Autodesk Inventor part; units mm, degrees
ref_plane "YZ Plane" through (0, 0, 0) normal (1, 0, 0) x (0, 1, 0)
ref_plane "XZ Plane" through (0, 0, 0) normal (0, 1, 0) x (-1, 0, 0)
ref_plane "XY Plane" through (0, 0, 0) normal (0, 0, 1) x (1, 0, 0)
sketch "Sketch1" plane through (0, 0, 0) normal (1, 0, 0) x (0, 1, 0)
  line L0 (-0.0645, -0.0614) -> (-0.0645, 12.6386) construction
  line L1 (-0.0645, 12.6386) -> (-0.0645, 25.3386) construction
  line L2 (-0.0645, -0.0614) -> (33.5905, -0.0614) construction
  line L3 (-0.0645, -0.0614) -> (33.5814, 17.8149) construction
  line L4 (33.5814, 17.8149) -> (33.5814, 30.5149) construction
  line L5 (33.5814, 30.5149) -> (33.5814, 43.2149) construction
  line L6 (-0.0645, -0.0614) -> (-0.0645, -25.4614) construction
  line L7 (-0.0645, -25.4614) -> (-0.0645, -50.8614) construction
  line L8 (-0.0645, -50.8614) -> (-0.0645, -88.9614) construction
  line L9 (-0.0645, -88.9614) -> (-0.0645, -127.0614) construction
  line L10 (-0.0645, -127.0614) -> (33.5905, -127.0614) construction
  line L11 (-0.0645, -127.0614) -> (33.5905, -144.9206) construction
  line L12 (-0.0645, -50.8614) -> (33.5905, -50.8614) construction
  line L13 (-0.0645, -50.8614) -> (33.5905, -68.7206) construction
  line L14 (33.5905, -68.7206) -> (33.5905, -81.4206) construction
  line L15 (33.5905, -81.4206) -> (33.5905, -94.1206) construction
  line L16 (33.5905, -144.9206) -> (33.5905, -106.8206) construction
  line L17 (33.5905, -106.8206) -> (96.5027, -106.8206) construction
  line L18 (33.5905, -144.9206) -> (56.4857, -106.8206) construction
  line L19 (33.5905, -68.7206) -> (56.4857, -106.8206) construction
  line L20 (-0.0645, -50.8614) -> (-0.0645, -63.5614) construction
  line L21 (-0.0645, -63.5614) -> (-0.0645, -76.2614) construction
  line L22 (33.5905, -0.0614) -> (67.2455, -0.0614) construction
  line L23 (67.2455, -0.0614) -> (33.5814, 17.8149) construction
  line L24 (67.2455, -0.0614) -> (67.2455, 25.3386) construction
  line L25 (67.2455, 25.3386) -> (67.2455, 25.3386) construction
  line L26 (67.2455, 25.3386) -> (73.5955, 25.3386) construction
  line L27 (67.2455, 25.3386) -> (60.8955, 25.3386) construction
  line L28 (-19.1145, -0.0711) -> (-19.1145, -127.0711)
  line L29 (-19.1145, -0.0711) -> (-19.1145, 32.0046)
  line L30 (-19.1145, 63.4289) -> (18.9855, 63.4289) construction
  line L31 (39.9379, -190.511) -> (19.05, -190.5323)
  line L32 (-19.05, -190.571) -> (-19.0726, -168.346) construction
  line L33 (-19.1145, 63.4289) -> (18.9855, 63.4289)
  line L34 (-19.1145, 63.4289) -> (-19.1145, 41.2039) construction
  line L35 (-19.05, -190.571) -> (-19.0726, -168.346)
  line L36 (-19.05, -190.571) -> (19.05, -190.5323) construction
  arc A0 (-11.2228, -178.4175) -> (19.05, -190.5323) centre (19.0055, -146.7627) ccw
  arc A1 (18.9855, 63.4289) -> (-10.4946, 51.0726) centre (22.5956, 13.4704) ccw
  line L37 (-19.1145, 41.2039) -> (-19.1145, 63.4289)
  line L38 (-19.081, -160.0737) -> (-19.1145, -127.0711)
  line L39 (19.05, -190.5323) -> (-19.05, -190.571)
  arc A2 (-10.4946, 51.0726) -> (-19.1145, 32.0046) centre (6.2855, 32.0046) ccw
  arc A3 (-19.081, -160.0737) -> (-11.2228, -178.4175) centre (6.319, -160.0479) ccw
  line L40 (82.55, -43.1133) -> (82.55, -47.5335)
  line L41 (82.55, -190.4677) -> (82.55, -154.3842)
  line L42 (82.55, 3.175) -> (82.55, 63.4289)
  line L43 (82.55, 63.4289) -> (18.9855, 63.4289)
  line L44 (19.05, -190.5323) -> (50.8, -190.5)
  line L45 (82.55, -190.4677) -> (82.55, -117.4427)
  arc A4 (59.4372, -181.357) -> (82.55, -117.4427) centre (-17.378, -117.4427) ccw
  arc A5 (39.9379, -190.511) -> (59.4372, -181.357) centre (39.9121, -165.1111) ccw
  line L46 (82.55, 63.4289) -> (82.55, -38.1711)
  line L47 (82.55, 63.4289) -> (114.3, 63.4289)
  line L48 (120.65, 57.0789) -> (120.65, 15.7647)
  arc A6 (108.6074, -5.8395) -> (95.5578, -16.5987) centre (141.4695, -58.9906) ccw
  arc A7 (84.9949, -32.2402) -> (82.55, -43.1133) centre (107.95, -43.1133) ccw
  arc A8 (108.6074, -5.8395) -> (120.65, 15.7647) centre (95.25, 15.7647) ccw
  arc A9 (120.65, 57.0789) -> (114.3, 63.4289) centre (114.3, 57.0789) ccw
  line L49 (82.55, -190.4677) -> (82.55, -79.4019)
  line L50 (82.55, -63.4677) -> (84.1375, -63.4677)
  line L51 (82.55, -117.4427) -> (82.55, -134.9348)
  line L52 (82.55, -117.4427) -> (82.55, -113.6327)
  line L53 (82.55, -63.4677) -> (88.9, -63.4677)
  line L54 (82.55, -63.4677) -> (82.55, -76.1677)
  line L55 (82.55, -63.4677) -> (82.55, -50.7677)
  arc A10 (88.9, -63.4677) -> (84.7021, -52.298) centre (76.3064, -61.827) ccw
  arc A11 (82.55, -47.5335) -> (84.7021, -52.298) centre (88.9, -47.5335) ccw
  arc A12 (84.7021, -74.6374) -> (82.55, -79.4019) centre (88.9, -79.4019) ccw
  line L56 (82.55, -63.4677) -> (84.1375, -63.4677)
  line L57 (84.1375, -63.4677) -> (84.1375, -139.6677)
  line L58 (82.55, -117.4427) -> (95.25, -139.6677)
  line L59 (95.25, -139.6677) -> (75.6405, -153.9552)
  line L60 (82.55, -63.4677) -> (77.47, -63.4677)
  line L61 (77.47, -63.4677) -> (77.47, -85.6927)
  line L62 (88.9, -63.4677) -> (88.9, -139.0447)
  line L63 (88.9, -63.4677) -> (88.8195, -33.8988)
  arc A13 (95.5578, -16.5987) -> (88.8195, -33.8988) centre (114.2194, -33.8296) ccw
  line L64 (33.5905, -144.9206) -> (48.1955, -144.9206)
  line L65 (48.1955, -144.9206) -> (48.1955, -119.5206)
  arc A14 (39.9379, -190.511) -> (88.9, -139.0447) centre (37.3696, -139.0447) ccw
  line L66 (84.1375, -139.6677) -> (48.1955, -139.6677)
  line L67 (48.1955, -139.6677) -> (48.1955, -119.5206)
  point P0 (82.55, -106.8206)
  point P1 (120.65, 63.4289)
  point P2 (120.65, -0.0711)
  point P3 (82.55, -148.9209)
  point P4 (88.7962, -25.3679)
  point P5 (88.8909, -60.1177)
  point P6 (44.795, -190.0373)
  dimension "d81" = 33.655
  dimension "d82" = 38.1
  dimension "d86" = 12.7
  dimension "d93" = 25.4
  dimension "d94" = 38.1
  dimension "d95" = 38.1
  dimension "d98" = 33.655
  dimension "d109" = 38.1
  dimension "d110" = 12.7
  dimension "d111" = 12.7
  dimension "d112" = 38.1
  dimension "d113" = 44.45
  dimension "d114" = 12.7
  dimension "d115" = 12.7
  dimension "d116" = 33.655
  dimension "d117" = 25.4
  dimension "d118" = 0
  dimension "d119" = 6.35
  dimension "d120" = 6.35
  dimension "d122" = 19.05
  dimension "d126" = 127
  dimension "d127" = 63.5
  dimension "d129" = 38.1
  dimension "d130" = 22.225
  dimension "d131" = 22.225
  dimension "d132" = 38.1
  dimension "d133" = 50.0888
  dimension "d134" = 25.4
  dimension "d135" = 25.4
  dimension "d137" = 31.75
  dimension "d138" = 73.025
  dimension "d139" = 25.4
  dimension "d140" = 101.6
  dimension "d141" = 38.1
  dimension "d142" = 25.4
  dimension "d143" = 6.35
  dimension "d144" = 62.4897
  dimension "d145" = 127
  dimension "d153" = 6.35
  dimension "d154" = 12.7
  dimension "d155" = 12.7
  dimension "d157" = 12.7
  dimension "d158" = 6.35
  dimension "d159" = 1.5875
  dimension "d160" = 76.2
  dimension "d161" = 5.08
  dimension "d162" = 22.225
  dimension "d163" = 38.1
  dimension "d164" = 25.4
  dimension "d166" = 25.4
extrude "Extrusion1" add sketch "Sketch1" along normal blind 1.5875 contours L29 A2 A1 L43 L47 A9 L48 A8 A6 A13 L63 L53 L57 A12 L49 A4 A5 A14 L31 A0 A3 L38 L28 | A5 A4 L59 L45 L41 A14 | L41 L45 L59 A14 | A4 L66 L45 L59 | L59 L45 L66 L57 L58 L62 A14 | A4 L45 L66 | L58 L57 L66 L45 | L49 A12 L57 L58 | L58 L57 L53 L62 | L63 A10
hole "Hole4" at (0, -0.0645, -0.0614) at (0, -0.0645, 12.6386) at (0, -0.0645, 25.3386) at (0, -0.0645, -127.0614) at (0, 33.5905, -144.9206) at (0, -0.0645, -50.8614) at (0, 33.5814, 43.2149) at (0, 33.5814, 30.5149) at (0, 33.5814, 17.8149) at (0, 33.5905, -68.7206) at (0, 33.5905, -81.4206) at (0, 33.5905, -94.1206) at (0, -0.0645, -63.5614) at (0, -0.0645, -76.2614) at (0, 56.4857, -106.8206) at (0, 60.8955, 25.3386) at (0, 73.5955, 25.3386) at (0, 48.1955, -119.5206) at (0, 84.1375, -63.4677) at (0, 77.47, -85.6927) at (0, 84.1375, -139.6677) direction (1, 0, 0) diameter 4.7625 end through all
properties part number "dtplate"
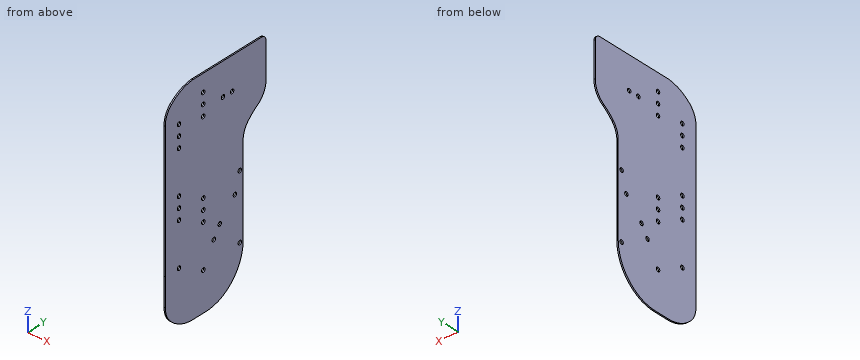
CAD build for the part. Positions are in the model's coordinates, mm. Give positions to 0.01 mm unless a question says otherwise; leave off trailing zeros. Order: outer loops, then holes, each group sorted by start corner. A loop starts at its lowest first (then second) coordinate and runs counter-clockwise, first axis right, second up. Notation, with made-up numbers: M 13.5,80 L 57.5,80 A18 cw 57.5,107 Z; hole C -14,-39 d8. An arc over 180 degrees is marked long. Put each result on its own line as item: value. Start each with the question number.
(1) Flat gauge pin, fed straight in: pin 1 Ø3 at (y, z) = (60.9, 25.34) entering from -X. Where does the tip first touch, or does it go through?
(2) Saw through at D-D, the plane z = -172. Write the cut outline in (x, y), then the cut area to 3 significant figures.
(3) Saw through at B-B, the plane y = 91.5. Write the cut outline in (x, z), then the cut area to 3 significant figures.
(4) Saw through at A-A, the plane z = 0. Write the cut outline in (x, y), then the cut area to 3 significant figures.
(5) Saw through at C-C, the plane x = 0.3. Give the number of separate pieces and of enclosed holes in the cut face, then the cut area to 3 significant figures.
(6) Drill centre lines: line 1 along Y through (x, z) = (1.15, 25); line 2 along Y through (x, z) = (1.2, -38); line 3 along Y through (x, z) = (1.2, 13). Where is each one in solid material? Low to high.
Check result:
1. pin 1: passes through
2. outline: M 0,-16.09 L 1.59,-16.09 L 1.59,76.98 L 0,76.98 Z
2. area: 148 mm2
3. outline: M 0,-22.47 L 1.59,-22.47 L 1.59,63.43 L 0,63.43 Z
3. area: 136 mm2
4. outline: M 0,-19.11 L 1.59,-19.11 L 1.59,-2.44 L 0,-2.44 Z; M 0,2.32 L 1.59,2.32 L 1.59,115.17 L 0,115.17 Z
4. area: 206 mm2
5. separate pieces: 1
5. enclosed holes: 21
5. area: 28,200 mm2
6. line 1: y = -19.11 to -2.42, 2.29 to 58.54, 63.25 to 71.24, 75.95 to 120.65
6. line 2: y = -19.11 to 88.83
6. line 3: y = -19.11 to -2.42, 2.29 to 120.5
